Autodesk Inventor part; units mm, degrees
ref_plane "ANBAU_XY" through (0, 0, 10.5) normal (0, 0, 1) x (1, 0, 0)
ref_plane "ANBAU_YZ" through (0, 0, 10.5) normal (1, 0, 0) x (0, 1, 0)
ref_plane "ANBAU_ZX" through (0, 0, 10.5) normal (0, 1, 0) x (0, 0, 1)
sketch "Sketch_1" plane through (0, 0, 0) normal (0, 0, 1) x (1, 0, 0)
  line L0 (15.7, 0) -> (-2.8, 0)
  arc A0 (0, 2.8) -> (-2.8, 0) centre (0, 0) ccw
  line L1 (0, 2.8) -> (4.8072, 2.8)
  line L2 (4.8072, 2.8) -> (5.5, 4)
  line L3 (5.5, 4) -> (12.4571, 4)
  line L4 (12.4571, 4) -> (13.2, 3.801)
  line L5 (13.2, 3.801) -> (13.2, 3.6938)
  line L6 (13.2, 3.6938) -> (13.4586, 3.6938)
  line L7 (13.4586, 3.6938) -> (13.6, 3.5524)
  line L8 (13.6, 3.5524) -> (13.6, 2.5)
  line L9 (13.6, 2.5) -> (14.13, 2.5)
  arc A1 (14.13, 2.5) -> (14.5, 2.87) centre (14.13, 2.87) ccw
  line L10 (14.5, 2.87) -> (14.5, 5.9)
  line L11 (14.5, 5.9) -> (14.8974, 5.9)
  arc A2 (15.0944, 5.7347) -> (14.8974, 5.9) centre (14.8974, 5.7) ccw
  line L12 (15.0944, 5.7347) -> (15.7, 2.3)
  line L13 (15.7, 2.3) -> (15.7, 0)
  line L14 (15.7, 0) -> (-2.8, 0)
revolve "Revolution1" add sketch "Sketch_1" angle 360 about axis through (15.7, 0, 0) along (-1, 0, 0)
sketch "Sketch_2" plane through (0, 0, 0) normal (1, 0, 0) x (0, 1, 0)
  line L0 (0, 0) -> (0, 10.5)
  line L1 (0, 10.5) -> (3.8, 10.5)
  line L2 (3.8, 10.5) -> (3.8, 10.1)
  line L3 (3.8, 10.1) -> (3.7, 10)
  line L4 (3.7, 10) -> (3.8, 9.9)
  line L5 (3.8, 9.9) -> (3.8, 8.5)
  line L6 (3.8, 8.5) -> (4, 8.5)
  line L7 (4, 8.5) -> (4.64, 8.1305)
  line L8 (4.64, 8.1305) -> (4.64, 5.3695)
  line L9 (4.64, 5.3695) -> (4, 5)
  line L10 (4, 5) -> (3.75, 5)
  line L11 (3.75, 5) -> (3.75, 4)
  line L12 (3.75, 4) -> (2.8, 3.05)
  line L13 (2.8, 3.05) -> (2.8, 0)
  line L14 (2.8, 0) -> (0, 0)
  line L15 (0, 0) -> (0, 10.5)
revolve "Revolution2" add sketch "Sketch_2" angle 360 about axis through (0, 0, 0) along (0, 0, 1)
sketch "Sketch_3" plane through (0, 0, 0) normal (1, 0, 0) x (0, 1, 0)
  line L0 (0, 10.5) -> (0, 13.5)
  line L1 (0, 13.5) -> (2.0095, 13.5)
  line L2 (2.0095, 13.5) -> (2.5, 13.0095)
  line L3 (2.5, 13.0095) -> (2.5, 10.5)
  line L4 (2.5, 10.5) -> (0, 10.5)
  line L5 (0, 10.5) -> (0, 13.5)
revolve "Revolution3" add sketch "Sketch_3" angle 360 about axis through (0, 0, 10.5) along (0, 0, 1)
thread "Thread1"
sketch "Sketch_11" plane through (15.7, 0, 0) normal (1, 0, 0) x (0, 0, -1)
  line L0 (-9.8, -5.658) -> (0, -11.3161)
  line L1 (0, -11.3161) -> (9.8, -5.658)
  line L2 (9.8, -5.658) -> (9.8, 5.658)
  line L3 (9.8, 5.658) -> (0, 11.3161)
  line L4 (0, 11.3161) -> (-9.8, 5.658)
  line L5 (-9.8, 5.658) -> (-9.8, -5.658)
  arc A0 (-1, 3.9) -> (-1, -3.9) centre (-1, 0) ccw
  line L6 (-1, -3.9) -> (1, -3.9)
  arc A1 (1, -3.9) -> (1, 3.9) centre (1, 0) ccw
  line L7 (1, 3.9) -> (-1, 3.9)
extrude "Extrusion1" cut sketch "Sketch_11" against normal blind 1.2
sketch "Sketch_5" plane through (0, 0, 0) normal (0, 1, 0) x (-1, 0, 0)
  line L0 (-15.7, 0) -> (0.85, 0)
  arc A0 (0, -0.85) -> (0.85, 0) centre (0, 0) ccw
  line L1 (0, -0.85) -> (-4.1, -0.85)
  line L2 (-4.1, -0.85) -> (-4.1, -2)
  line L3 (-4.1, -2) -> (-15.4, -2)
  arc A1 (-15.4, -2) -> (-15.7, -2.3) centre (-15.4, -2.3) ccw
  line L4 (-15.7, -2.3) -> (-15.7, 0)
  line L5 (-15.7, 0) -> (0.85, 0)
sketch "Sketch_15" plane through (0, 0, 0) normal (0, 1, 0) x (-1, 0, 0)
  line L0 (3.75, -1) -> (3.75, 4)
  line L1 (3.75, 4) -> (-5.5, 4)
  line L2 (-5.5, 4) -> (-5.5, -4)
  line L3 (-5.5, -4) -> (0.75, -4)
  arc A0 (0.75, -4) -> (3.75, -1) centre (0.75, -1) ccw
extrude "Extrusion2" add sketch "Sketch_15" along normal mid plane 1
sketch "Sketch_6" plane through (0, 0, 0) normal (1, 0, 0) x (0, 1, 0)
  line L0 (0, 0) -> (0, 13.5)
  line L1 (0, 13.5) -> (0.85, 13.5)
  line L2 (0.85, 13.5) -> (0.85, 0)
  line L3 (0.85, 0) -> (0, 0)
  line L4 (0, 0) -> (0, 13.5)
revolve "Revolution4" cut sketch "Sketch_6" angle 360 about axis through (0, 0, 0) along (0, 0, 1)
revolve "Revolution5" cut sketch "Sketch_5" angle 360 about axis through (15.7, 0, 0) along (-1, 0, 0)
sketch "Sketch_9" plane through (0, 0, 10.5) normal (0, 0, 1) x (1, 0, 0)
  line L0 (-8, -8) -> (8, -8)
  line L1 (8, -8) -> (8, 8)
  line L2 (8, 8) -> (-8, 8)
  line L3 (-8, 8) -> (-8, -8)
  line L4 (-4.6188, 0) -> (-2.3094, -4)
  line L5 (-2.3094, -4) -> (2.3094, -4)
  line L6 (2.3094, -4) -> (4.6188, 0)
  line L7 (4.6188, 0) -> (2.3094, 4)
  line L8 (2.3094, 4) -> (-2.3094, 4)
  line L9 (-2.3094, 4) -> (-4.6188, 0)
extrude "Extrusion3" cut sketch "Sketch_9" against normal blind 6.0556
ref_plane "ANBAU_XY" through (0, 0, 10.5) normal (0, 0, 1) x (1, 0, 0)
ref_plane "ANBAU_YZ" through (0, 0, 10.5) normal (1, 0, 0) x (0, 1, 0)
ref_plane "ANBAU_ZX" through (0, 0, 10.5) normal (0, 1, 0) x (0, 0, 1)
ref_plane "ANBAU_STD_XY" through (0, 0, 10.5) normal (0, 0, -1) x (1, 0, 0)
ref_plane "ANBAU_STD_YZ" through (0, 0, 10.5) normal (1, 0, 0) x (0, -1, 0)
ref_plane "ANBAU_STD_ZX" through (0, 0, 10.5) normal (0, -1, 0) x (0, 0, -1)
ref_plane "CPV_XY" through (0, 0, 10.5) normal (0, 0, -1) x (1, 0, 0)
ref_plane "CPV_YZ" through (0, 0, 10.5) normal (1, 0, 0) x (0, -1, 0)
ref_plane "CPV_ZX" through (0, 0, 10.5) normal (0, -1, 0) x (0, 0, -1)
ref_plane "FDT_MOUNT_XY" through (0, 0, 10.5) normal (0, 0, 1) x (0, 1, 0)
ref_plane "FDT_MOUNT_YZ" through (0, 0, 10.5) normal (0, 1, 0) x (-1, 0, 0)
ref_plane "FDT_MOUNT_ZX" through (0, 0, 10.5) normal (-1, 0, 0) x (0, 0, 1)
ref_plane "FDT_SCHLAUCH_XY" through (4.1, 0, 0) normal (1, 0, 0) x (0, 0, -1)
ref_plane "FDT_SCHLAUCH_YZ" through (4.1, 0, 0) normal (0, 0, -1) x (0, 1, 0)
ref_plane "FDT_SCHLAUCH_ZX" through (4.1, 0, 0) normal (0, 1, 0) x (1, 0, 0)
properties part number "153333 QSML-M5-4"
The model under review builds one solid part; all positions refer to its coordinate system, in mm. A direction names the side the tool comes from. Give positions to 0.01 mm unless a question says otherwise; leave off trailing zeros. Loops run counter-clockwise (first coordinate to the right, second up) from the corner with the lowest first, then second, coordinate; pieces in that order, holes last. Notation, with made-up numbers: (3, 34.5) -> (17, 34.5) arc R11 ccw to (17, 53.5) -> close; hole circle Ø6 at (-38.5, -29). An arc over 180 degrees is marked (long way). Use CSV: the item, a comma, the result in double quotes.
1. For P1, Ø2, axis at x = 7.5, y = 2, coming from the -Z side; P2, Ø1.4, axis at x = 3.5, z = 3.5, coming from the -Y side; P3, Ø0.7, axis at x = 15, z = 0.5, coming from the +Y side, all flat-tipped, find the tip position at first contact; note any pin that passes through.
Result:
P1,"stops at z = -3.87"
P2,"stops at y = -2.24"
P3,"stops at y = 3.9"
2. Machinability: for faces 1 (the face through (15, 3.9, 0)), 2 (the face through (-0.83, -0.18, 6.66)), 3 (the face through (13.87, -0.54, -2.44)), which of the approach directions +Z, -Z, +X, -X, +Y, -Y give a long, thin tool a straight path to every point of the face, cutting with its end or side? Answer none if there is none.
Result:
face 1,"+Z, -Z, +X, +Y"
face 2,"+Z"
face 3,"none"
3. To check wall thickness, follow probe 1 along Y at (x, z) = (1.35, 0); probe 2 along Z at (x, y) = (2.05, 0); probe 3 along Z at (x, y) = (3.05, 0). State the ranges of each line that lie inside material, in increasing order. Write a range as from..to.
Result:
probe 1,"y = -2.8..-0.85, 0.85..2.8"
probe 2,"z = -4..-0.85, 0.85..13.46"
probe 3,"z = -4..-0.85, 0.85..10.5"
4. Consider section A-A, the plane x = 6. Write out the cut boundary in (y, z), then the cut area to 3 significant figures.
Result:
outline,"circle Ø8 at (0, 0); hole circle Ø4 at (0, 0)"
area,"37.7 mm²"
5. The part is to be moulded in two halves that separate along Z. For faces 4 (the face through (-4.196, -0.01, 8.387)), 5 (the face through (4.93, -3.01, 0.06)), 6 (the face through (5, 0, 4)), 7 (the face through (14.5, -3, -1)), say which applies: +Z half, -Z half, draft (parallel to the pull), parting line (faces both ways), or undercut.
Result:
face 4,"+Z half"
face 5,"parting line"
face 6,"undercut"
face 7,"draft"
